```python
from build123d import *

# Parameters (mm, degrees)
BOSS_EXTRUDE1_DEPTH = 5
SKETCH3_W           = 8
SKETCH3_H           = 4
BOSS_EXTRUDE2_DEPTH = 3
FILLET1_START       = -3.841593316
FILLET1_DEPTH       = 8


with BuildPart() as part:
    # Sketch1 → Boss-Extrude1 (new body)
    with BuildSketch(Plane(origin=(0, 0, 0), x_dir=(1, 0, 0), z_dir=(0, 1, 0))):
        with BuildLine():
            Line((-30, 0), (30, 0))
            ThreePointArc((30, 0), (0, 30), (-30, 0))
        make_face()
    extrude(amount=BOSS_EXTRUDE1_DEPTH)

    # Sketch3 → Boss-Extrude2 (add)
    with BuildSketch(Plane(origin=(0, 5, 0), x_dir=(1, 0, 0), z_dir=(0, 1, 0))):
        with Locations((0.158406684, 24.731666579)):
            Rectangle(SKETCH3_W, SKETCH3_H)
    extrude(amount=BOSS_EXTRUDE2_DEPTH)

    # Fillet1: read off the stored shape, not the designer's step
    # Fillet1 outline → Fillet1 (cut)
    with BuildSketch(Plane.YZ.offset(FILLET1_START)):
        with BuildLine():
            Line((8, -22.731666579), (5, -22.731666579))
            add(Edge.make_bspline(
                [(5, -22.731666579), (8, -23.506263249), (8, -26.604649926)],
                knots=[0, 0, 0, 1, 1, 1], degree=2, weights=[1, 0.057495957, 1]))
            Line((8, -26.604649926), (8, -22.731666579))
        make_face()
    extrude(amount=FILLET1_DEPTH, mode=Mode.SUBTRACT)


solid = part.part
```
Geometry check sheet. Reference: the model listing, model coordinates, mm. A direction names the side the tool comes from. Give positions to 0.01 mm unless a question says otherwise; leave off trailing zeros. Loops run counter-clockwise (first coordinate to the right, second up) from the corner with the lowest first, then second, coordinate; pieces in that order, holes last. Notation, with made-up numbers: (70.25, 25) - (113.25, 25) arc R37 cw to (113.25, 64) - close; hole circle Ø11 at (-26.5, -28). An arc over 180 degrees is marked (long way). Use CSV: the item, a comma, the result in double quotes. Start each with the question number.
Q1. Section check C-C, the plane z = -10. Record the cut outline in (x, y), and give its area (3 significant figures).
Q2. Scan lines: probe 1 along Y at (x, z) = (-1, -17); probe 2 along X at (y, z) = (6.5, -25.75); probe 3 along Z at (x, y) = (-7, 0.75). Record each from-to range of solid material in increasing order. Write a range as from..to.
Q3. Access from +Z, -Z, +X, -X, +Y, -Y to the whole of each face (thin tool, end or side, straight path). Record for faces 1 (the face through (4.158, 6, -25)), 2 (the face through (0, 2, 0)), 3 (the face through (0, 6, -26.732)), 4 (the face through (-3.842, 6, -25)).
Q4. Section check A-A, the plane x = 24. Record the cut outline in (y, z).
Q5. Go/stop test with flat-tipped pins: pin 1 Ø3.5 at (y, z) = (6, -25.5) entering from +X; pin 2 Ø4 at (x, y) = (-14, 6) entering from -Z; pin 3 Ø2.5 at (x, y) = (-1, 6) entering from -Z. Record where each tip stops, or that it passes through.
Q6. Section check B-B, the plane y = 0.75. Record the cut outline in (x, z).
Findings below:
1,outline,"(-28.28, 0) - (28.28, 0) - (28.28, 5) - (-28.28, 5) - close"
1,area,"283 mm^2"
2,probe 1,"y = 0..5"
2,probe 2,"x = -3.84..4.16"
2,probe 3,"z = -29.17..0"
3,face 1,"+Z, -Z, +X, +Y"
3,face 2,"+Z, +X, -X, +Y, -Y"
3,face 3,"-Z, +X, -X, +Y"
3,face 4,"+Z, -Z, -X, +Y"
4,outline,"(0, -18) - (5, -18) - (5, 0) - (0, 0) - close"
5,pin 1,"stops at x = 17.91"
5,pin 2,"stops at z = -27.38"
5,pin 3,"stops at z = -30"
6,outline,"(-30, 0) arc R30 ccw to (30, 0) - close"
